Autodesk Inventor part; units mm, degrees
ref_plane "YZ Plane" through (0, 0, 0) normal (1, 0, 0) x (0, 1, 0)
ref_plane "XZ Plane" through (0, 0, 0) normal (0, 1, 0) x (-1, 0, 0)
ref_plane "XY Plane" through (0, 0, 0) normal (0, 0, 1) x (1, 0, 0)
sketch "Sketch1" plane through (0, 0, 0) normal (0, 1, 0) x (-1, 0, 0)
  line L0 (22.75, -10.36) -> (7.75, -10.36)
  line L1 (7.75, -10.36) -> (-0.1031, 0)
  circle A0 centre (4.34, -10.36) radius 1
  line L2 (22.75, 10.36) -> (7.75, 10.36)
  circle A1 centre (12.64, 0) radius 9.6 construction
  line L3 (22.75, 12.36) -> (22.75, -12.36)
  circle A2 centre (4.34, 10.36) radius 1
  line L4 (7.75, 10.36) -> (-0.1031, 0)
  line L5 (26.25, 19) -> (26.25, -19)
  line L6 (22.75, -12.36) -> (-22.75, -12.36)
  line L7 (22.75, 0) -> (-22.75, 0) construction
  line L8 (26.25, -19) -> (-28.75, -19)
  line L9 (26.25, -19) -> (-28.75, 19) construction
  line L10 (-28.75, -19) -> (26.25, 19) construction
  line L11 (-22.75, 12.36) -> (22.75, 12.36)
  line L12 (-28.75, 19) -> (26.25, 19)
  line L13 (-28.75, -19) -> (-28.75, 19)
  circle A3 centre (-16.36, 10.25) radius 1
  line L14 (-22.75, -12.36) -> (-22.75, 12.36)
  circle A4 centre (-16.36, -10.25) radius 1
  point P0 (0, 0)
  point P1 (-1.25, 0)
  point P2 (0, 0)
  point P3 (22.75, -10.36)
  dimension "d0" = 55
  dimension "d1" = 38
  dimension "d2" = 45.5
  dimension "d3" = 24.72
  dimension "d4" = 2
  dimension "d6" = 18.41
  dimension "d7" = 20.5
  dimension "d8" = 19.2
  dimension "d9" = 10.11
  dimension "d10" = 13
  dimension "d11" = 15
  dimension "d12" = 3.5
  dimension "d13" = 2
  dimension "d14" = 3.41
  dimension "d51" = 20.7
extrude "Extrusion1" add sketch "Sketch1" along normal mid plane 1 contours L3 L6 L14 L11 L2 L4 L1 L0 | L5 L8 L13 L12
extrude "Extrusion2" add sketch "Sketch1" along normal blind 35 contours L5 L8 L13 L12
fillet "Fillet1" radius 3 8 edges at (1.25, -0.5, -19) (28.75, -0.5, 0) (1.25, -0.5, 19) (-26.25, -0.5, 0) (28.75, 17.25, -19) (28.75, 17.25, 19) (-26.25, 17.25, 19) (-26.25, 17.25, -19)
sketch "Sketch3" plane through (-23.25, 35, 19) normal (0, 0, 1) x (1, 0, 0)
  line L0 (46.5, -34.5) -> (46.5, 0)
  circle A0 centre (46.5, -17.75) radius 1.5
  circle A1 centre (46.5, -10.75) radius 1.5
  circle A2 centre (46.5, -3.75) radius 1.5
  circle A3 centre (32.5, -17.75) radius 1.5
  circle A4 centre (32.5, -10.75) radius 1.5
  circle A5 centre (32.5, -3.75) radius 1.5
  line L1 (52, -32.5) -> (52, 0)
  line L2 (0, 0) -> (49, 0)
  dimension "d23" = 7
  dimension "d26" = 14
  dimension "d52" = 5.5
  dimension "d53" = 3.75
hole "Hole1" at (23.25, 17.25, 19) at (9.25, 17.25, 19) at (9.25, 24.25, 19) at (23.25, 24.25, 19) at (23.25, 31.25, 19) at (9.25, 31.25, 19) direction (0, 0, -1) diameter 2.459 depth 5.8 tip angle 118 counterbore diameter 3.9 counterbore depth 3
sketch "Sketch6" plane through (0, 35, 0) normal (0, 1, 0) x (1, 0, 0)
  line L0 (25.75, 19) -> (-23.25, 19)
  line L1 (28.75, -16) -> (28.75, 16)
  point P0 (0, 0)
  point P1 (16.25, 15.68)
  dimension "d64" = 3.32
  dimension "d65" = 12.5
hole "Hole2" at (16.25, 35, -15.68) direction (0, -1, 0) diameter 2.459 depth 6 tip angle 118 counterbore diameter 3.9 counterbore depth 3.8
properties part number "basket" material "PCTG 20%"
Can you work these out from the model? Positions are in its coordinate system, mm. A direction names the side the tool comes from. Give positions to 0.01 mm unless a question says otherwise; leave off trailing zeros. Order: outer loops, then holes, each group sorted by start corner. A loop starts at its lowest first (then second) coordinate and runs counter-clockwise, first axis right, second up. Notation, with made-up numbers: (57.25, 15.25) - (78.25, 15.25) arc R3 cw to (78.25, 19.25) - close; hole circle Ø10 at (3.25, -4.75). An arc over 180 degrees is marked (long way). Write each question's results on one line, items separated by ' | '.
1) On a 3-axis mill with a long thin cutter (end or side, diameter ignored), from which of +Z, -Z, +X, -X, +Y, -Y can I reach the whole of each face in a straight line? I mean faces 4 (the face through (9.2, 19.2, 17.5)), 5 (the face through (28.75, 19, 0)), 6 (the face through (-22.75, 17, 0)). Say none if no direction works.
Final values:
face 4: +Z | face 5: +Z, -Z, +X, +Y, -Y | face 6: +Y
2) Suppose I cut it at B-B, the plane y = 9. Write out the boundary of the cut face in (x, z).
Final values:
outline: (-26.25, -16) arc R3 ccw to (-23.25, -19) - (25.75, -19) arc R3 ccw to (28.75, -16) - (28.75, 16) arc R3 ccw to (25.75, 19) - (-23.25, 19) arc R3 ccw to (-26.25, 16) - close; hole (-22.75, -12.36) - (22.75, -12.36) - (22.75, 12.36) - (-22.75, 12.36) - close
3) Please list where these lines run through material, in increasing order: line 1 along Y through (x, z) = (23.25, 14.9); line 2 along Z through (x, y) = (16.25, 34.25); line 3 along X through (y, z) = (27.5, 1.5). Write a range as [from, to].
Final values:
line 1: y = [-0.5, 16.02], [18.48, 23.02], [25.48, 30.02], [32.48, 35] | line 2: z = [-19, -17.63], [-13.73, -12.36], [12.36, 19] | line 3: x = [-26.25, -22.75], [22.75, 28.75]
4) Suppose I cut it at C-C, the plane z = 5.5. Write out the boundary of the cut face in (x, y).
Final values:
outline: (-26.25, 2.5) arc R3 ccw to (-23.25, -0.5) - (-22.75, -0.5) - (-22.75, 35) - (-26.25, 35) - close; (-4.07, -0.5) - (25.75, -0.5) arc R3 ccw to (28.75, 2.5) - (28.75, 35) - (22.75, 35) - (22.75, 0.5) - (-4.07, 0.5) - close
5) If we mould it in two halves opening along X, with no side actions, what happens to faces 1 (the face through (15.406, -0.007, 9.95)), 2 (the face through (1, 19, -19)), 3 (the face through (-26.25, 19, 0))? For each: pulls with the +X half, pulls with the -X half, needs draft (parallel to the pull), parting line crosses it, or undercut.
Final values:
face 1: undercut | face 2: needs draft | face 3: pulls with the -X half
6) I'm going to push flat-ended pins straight in: pin 1 Ø1 at (x, z) = (16.5, 0.5) entering from +Y; pin 2 Ø3 at (x, y) = (23.25, 24.25) entering from +Z; pin 3 Ø2 at (x, y) = (23.25, 17.25) entering from +Z. Where does each tip first touch, or does it pass through?
Final values:
pin 1: stops at y = 0.5 | pin 2: stops at z = 16 | pin 3: stops at z = 13.06
7) Suppose I cut it at A-A, the plane x = -20. Write out the boundary of the cut face in (y, z), then the cut area to 3 significant figures.
Final values:
outline: (-0.5, -16) arc R3 ccw to (2.5, -19) - (35, -19) - (35, -12.36) - (0.5, -12.36) - (0.5, -10.36) - (-0.5, -10.36) - close; (-0.5, 10.36) - (0.5, 10.36) - (0.5, 12.36) - (35, 12.36) - (35, 19) - (2.5, 19) arc R3 ccw to (-0.5, 16) - close | area: 472 mm^2
8) Suppose I cut it at D-D, the plane x = 2. Write out the boundary of the cut face in (y, z), then the cut area to 3 significant figures.
Final values:
outline: (-0.5, -16) arc R3 ccw to (2.5, -19) - (35, -19) - (35, -12.36) - (0.5, -12.36) - (0.5, 12.36) - (35, 12.36) - (35, 19) - (2.5, 19) arc R3 ccw to (-0.5, 16) - close | area: 492 mm^2
